The model under review builds one solid part; all positions refer to its coordinate system, in mm. A direction names the side the tool comes from. Coordinates: 2 decimals unless noted, no trailing zeros. Order: outer loops, then holes, each group sorted by start corner. A loop starts at its lowest first (then second) coordinate and runs counter-clockwise, first axis right, second up. Notation, with made-up numbers: (-24.5, -31.75) -> (-17.5, -31.75) arc R19 ccw to (-17.5, -2.75) -> close; hole circle Ø1 at (15.5, -25.75). An arc over 180 degrees is marked (long way). Use one line per item in the form item = value.
from build123d import *

# Parameters (mm, degrees)
SKETCH1_W               = 355.6
SKETCH1_H               = 406.4
BOSS_EXTRUDE1_DEPTH     = 15.875
SKETCH2_R               = 6.35
CUT_EXTRUDE1_DEPTH      = 16.875
MIRROR2_COPY_1_SKETCH_R = 6.35
MIRROR2_COPY_1_DEPTH    = 16.875
SKETCH3_R               = 14.2875
SKETCH3_R_2             = 4.064
CUT_EXTRUDE2_DEPTH      = 16.875
SKETCH4_R               = 25.4
CUT_EXTRUDE3_DEPTH      = 12.7
SKETCH5_R               = 6.35
CUT_EXTRUDE4_DEPTH      = 8.89


with BuildPart() as part:
    # Sketch1 → Boss-Extrude1 (new body)
    with BuildSketch(Plane(origin=(0, 0, 0), x_dir=(1, 0, 0), z_dir=(0, 1, 0))):
        Rectangle(SKETCH1_W, SKETCH1_H)
    extrude(amount=BOSS_EXTRUDE1_DEPTH)

    # Sketch2 → Cut-Extrude1 (cut, through all)
    with BuildSketch(Plane(origin=(0, 15.875, 0), x_dir=(1, 0, 0), z_dir=(0, 1, 0))):
        with Locations((-152.4, 177.8)):
            Circle(SKETCH2_R)
    cut_extrude1 = extrude(amount=-CUT_EXTRUDE1_DEPTH, mode=Mode.SUBTRACT)

    # Mirror1: Cut-Extrude1 across plane
    add(cut_extrude1.mirror(Plane.ZY), mode=Mode.SUBTRACT)

    # Mirror2: Cut-Extrude1 across plane
    add(cut_extrude1.mirror(Plane(origin=(0, 0, 0), x_dir=(1, 0, 0), z_dir=(0, 0, -1))), mode=Mode.SUBTRACT)

    # Mirror2 copy 1 sketch → Mirror2 copy 1 (cut, through all)
    with BuildSketch(Plane(origin=(0, 15.875, 0), x_dir=(-1, 0, 0), z_dir=(0, 1, 0))):
        with Locations((-152.4, 177.8)):
            Circle(MIRROR2_COPY_1_SKETCH_R)
    extrude(amount=-MIRROR2_COPY_1_DEPTH, mode=Mode.SUBTRACT)

    # Sketch3 → Cut-Extrude2 (cut, through all)
    with BuildSketch(Plane(origin=(0, 15.875, 0), x_dir=(1, 0, 0), z_dir=(0, 1, 0))):
        with Locations((0, 66.675)):
            Circle(SKETCH3_R)
        with Locations((-63.5, -22.225)):
            Circle(SKETCH3_R_2)
        with Locations((63.5, -22.225)):
            Circle(SKETCH3_R_2)
        with Locations((44.45, -107.95)):
            Circle(SKETCH3_R_2)
        with Locations((-44.45, -107.95)):
            Circle(SKETCH3_R_2)
        with Locations((-31.75, 98.425)):
            Circle(SKETCH3_R_2)
        with Locations((-31.75, 34.925)):
            Circle(SKETCH3_R_2)
        with Locations((31.75, 98.425)):
            Circle(SKETCH3_R_2)
        with Locations((31.75, 34.925)):
            Circle(SKETCH3_R_2)
    extrude(amount=-CUT_EXTRUDE2_DEPTH, mode=Mode.SUBTRACT)

    # Sketch4 → Cut-Extrude3 (cut)
    with BuildSketch(Plane(origin=(0, 15.875, 0), x_dir=(1, 0, 0), z_dir=(0, 1, 0))):
        with Locations((0, 66.675)):
            Circle(SKETCH4_R)
    extrude(amount=-CUT_EXTRUDE3_DEPTH, mode=Mode.SUBTRACT)

    # Sketch5 → Cut-Extrude4 (cut)
    with BuildSketch(Plane.XZ):
        with Locations((-31.75, -98.425)):
            Circle(SKETCH5_R)
        with Locations((31.75, -98.425)):
            Circle(SKETCH5_R)
        with Locations((31.75, -34.925)):
            Circle(SKETCH5_R)
        with Locations((-31.75, -34.925)):
            Circle(SKETCH5_R)
        with Locations((-63.5, 22.225)):
            Circle(SKETCH5_R)
        with Locations((63.5, 22.225)):
            Circle(SKETCH5_R)
        with Locations((44.45, 107.95)):
            Circle(SKETCH5_R)
        with Locations((-44.45, 107.95)):
            Circle(SKETCH5_R)
    extrude(amount=-CUT_EXTRUDE4_DEPTH, mode=Mode.SUBTRACT)


solid = part.part
Item 1: Clearance check with a flat-ended pin moving along its axis: pin 1 (10 mm diameter, centred on x = 31.75, z = -98.425, fed in from -Y). State where the tip first meets the part, or that it passes through.
Results found:
pin_1 = 8.89
Item 2: Draft analysis for pull direction X (two halves, no side actions). For faces 3 (the face through (-2, 8, 203.2)), 4 (the face through (-40.696, 12.431, 109.507)), state which applies: released by +X, released by -X, zero draft, split by the parting line, or undercut.
Results found:
face_3 = zero draft
face_4 = undercut
Item 3: We need section B-B (z = -46.5). Write out the cut boundary in (x, y) (3 decimals), plus the area to 3 significant figures.
Results found:
outline = (-177.8, 0) -> (177.8, 0) -> (177.8, 15.875) -> (15.431, 15.875) -> (15.431, 3.175) -> (-15.431, 3.175) -> (-15.431, 15.875) -> (-177.8, 15.875) -> close
area = 5,250 mm²
Item 4: To check wall thickness, follow L1, parallel to Z at x = 153.5, y = 6; L2, parallel to X at y = 2.75, z = -177.5; L3, parallel to Z at x = -44.45, y = 2.25. State the ranges of each line that lie inside material, in increasing order. Write a range as from..to.
Results found:
L1 = -203.2..-184.05, -171.55..171.55, 184.05..203.2
L2 = -177.8..-158.74, -146.06..146.06, 158.74..177.8
L3 = -203.2..101.6, 114.3..203.2
Item 5: Tool access review of faces 1 (the face through (-32.279, 12.431, -38.954)), 2 (the face through (47.38, 4.383, 102.316)): name each direction out of +Z, -Z, +X, -X, +Y, -Y from which nothing blocks a thin tool from reaching the whole face with its end or side.
Results found:
face_1 = +Y, -Y
face_2 = -Y
Item 6: We need section A-A (y = 12). State how many separate pieces and enclosed holes the cut face has, plus the area to 3 significant figures.
Results found:
separate_pieces = 1
enclosed_holes = 13
area = 142,000 mm²
